CAD build for the part. Positions are in the model's coordinates, mm. A direction names the side the tool comes from. Coordinates: 2 decimals unless noted, no trailing zeros. Loops run counter-clockwise (first coordinate to the right, second up) from the corner with the lowest first, then second, coordinate; pieces in that order, holes last.
1) Which spindle directions (+Z, -Z, +X, -X, +Y, -Y) get a long thin tool onto all of the face, cutting with end or side? Do faces 1 (the flat face through (-1, -4, 1)), 2 (the cylindrical face through (-50.56, -3.26, 22.64)), 3 (the cylindrical face through (23.4, 1, -77.3)). Say none if no direction does.
2) Wall check: line 1 along X through (y, z) = (61.9, 87.42); line 2 along Z through (x, y) = (-12.5, 18.5); line 3 along Z through (x, y) = (-86.5, 63.55). Give the ranges that are in metal, low to high.
3) Pin check, flat tips, straight feed: pin 1 Ø0.8 at (x, z) = (-57, -70) entering from +Y; pin 2 Ø0.8 at (x, z) = (-25, -25.5) entering from -Y; pin 3 Ø0.6 at (y, z) = (28.5, -92) entering from -X. Stop position of each tip, or through.
4) Saw through at A-A, the plane y = 51. Write the cut outline in (x, z).
5) Saw through at B-B, the plane x = -4.5. Write the cut outline in (y, z).
6) Saw through at D-D, the plane x = 38.5. Write the cut outline in (y, z).
7) Two-plate mould, pull along Z, no slides. Class faces 4 (the flat face through (-1, 39, -92.92)), 5 (the cylindrical face through (-89.15, 30.98, 89.91)), 6 (the flat face through (86, 33, 83.92)): +Z half, -Z half, draft (parallel to the pull), parting line (faces both ways), or undercut.
8) Saw through at C-C, the plane z = 45. Write the cut outline in (x, y), and give its area (3 significant figures).
```python
from build123d import *

# Parameters (mm, degrees)
SKETCH1_W           = 184
SKETCH1_H           = 185.84
SKETCH1_W_2         = 180
SKETCH1_H_2         = 181.84
SKETCH1_W_3         = 7
SKETCH1_H_3         = 7
BOSS_EXTRUDE1_DEPTH = 65
SKETCH2_W           = 184
SKETCH2_H           = 185.84
BOSS_EXTRUDE2_DEPTH = 4
CUT_EXTRUDE1_REACH  = 187.84
SKETCH3_W           = 21.03
SKETCH3_H           = 16.02
CUT_EXTRUDE4_REACH  = 186
SKETCH4_R           = 1.75
SKETCH4_R_2         = 8.065
SKETCH4_W           = 4.5
SKETCH4_H           = 8.3
CUT_EXTRUDE3_REACH  = 187.84
SKETCH6_W           = 8.3
SKETCH6_H           = 4.5
SKETCH6_W_2         = 21.85
SKETCH6_H_2         = 30.2
SKETCH8_R           = 3.4
SKETCH8_R_2         = 1.4
SKETCH8_R_3         = 2.9
SKETCH8_R_4         = 0.9
BOSS_EXTRUDE3_DEPTH = 2
SKETCH8_3_R         = 2.14
BOSS_EXTRUDE4_DEPTH = 4
CUT_EXTRUDE5_REACH  = 6
SKETCH8_4_R         = 1.25
SKETCH9_R           = 2.25
CUT_EXTRUDE6_DEPTH  = 1.5
SKETCH10_R          = 1.4
CUT_EXTRUDE7_DEPTH  = 4
FILLET1_R           = 10
FILLET2_R           = 2
SKETCH11_R          = 1.4
CUT_EXTRUDE8_DEPTH  = 2.5


with BuildPart() as part:
    # Sketch1 → Boss-Extrude1 (new body)
    with BuildSketch(Plane(origin=(0, 0, 0), x_dir=(1, 0, 0), z_dir=(0, 1, 0))):
        Rectangle(SKETCH1_W, SKETCH1_H)
        Rectangle(SKETCH1_W_2, SKETCH1_H_2, mode=Mode.SUBTRACT)
        with Locations((-86.5, 87.42)):
            Rectangle(SKETCH1_W_3, SKETCH1_H_3)
        with Locations((86.5, 87.42)):
            Rectangle(SKETCH1_W_3, SKETCH1_H_3)
        with Locations((-86.5, -87.42)):
            Rectangle(SKETCH1_W_3, SKETCH1_H_3)
        with Locations((86.5, -87.42)):
            Rectangle(SKETCH1_W_3, SKETCH1_H_3)
    extrude(amount=BOSS_EXTRUDE1_DEPTH)

    # Sketch2 → Boss-Extrude2 (add)
    with BuildSketch(Plane.XZ):
        Rectangle(SKETCH2_W, SKETCH2_H)
    extrude(amount=BOSS_EXTRUDE2_DEPTH)

    # Sketch3 → Cut-Extrude1 (cut, up to next)
    with BuildSketch(Plane(origin=(0, 0, -92.92), x_dir=(-1, 0, 0), z_dir=(0, 0, -1)), mode=Mode.PRIVATE) as cut_extrude1_sk1:
        with Locations((0, 30.5)):
            Rectangle(SKETCH3_W, SKETCH3_H)
    cut_extrude1_tool1 = extrude(cut_extrude1_sk1.sketch, amount=-CUT_EXTRUDE1_REACH, mode=Mode.PRIVATE) & part.part
    add(cut_extrude1_tool1.solids().sort_by_distance((0, 30.5, -92.92))[0], mode=Mode.SUBTRACT)

    # Sketch4 → Cut-Extrude4 (cut, up to next)
    with BuildSketch(Plane(origin=(92, 0, 0), x_dir=(0, 0, -1), z_dir=(1, 0, 0)), mode=Mode.PRIVATE) as cut_extrude4_sk1:
        with Locations((-54.360232663, 46.940232663)):
            Circle(SKETCH4_R)
    cut_extrude4_tool1 = extrude(cut_extrude4_sk1.sketch, amount=-CUT_EXTRUDE4_REACH, mode=Mode.PRIVATE) & part.part
    add(cut_extrude4_tool1.solids().sort_by_distance((92, 46.940233, 54.360233))[0], mode=Mode.SUBTRACT)
    # Sketch4 → Cut-Extrude4 (cut, up to next)
    with BuildSketch(Plane(origin=(92, 0, 0), x_dir=(0, 0, -1), z_dir=(1, 0, 0)), mode=Mode.PRIVATE) as cut_extrude4_sk2:
        with Locations((-21.479767337, 14.059767337)):
            Circle(SKETCH4_R)
    cut_extrude4_tool2 = extrude(cut_extrude4_sk2.sketch, amount=-CUT_EXTRUDE4_REACH, mode=Mode.PRIVATE) & part.part
    add(cut_extrude4_tool2.solids().sort_by_distance((92, 14.059767, 21.479767))[0], mode=Mode.SUBTRACT)
    # Sketch4 → Cut-Extrude4 (cut, up to next)
    with BuildSketch(Plane(origin=(92, 0, 0), x_dir=(0, 0, -1), z_dir=(1, 0, 0)), mode=Mode.PRIVATE) as cut_extrude4_sk3:
        with Locations((52.92, 30.5)):
            Circle(SKETCH4_R_2)
    cut_extrude4_tool3 = extrude(cut_extrude4_sk3.sketch, amount=-CUT_EXTRUDE4_REACH, mode=Mode.PRIVATE) & part.part
    add(cut_extrude4_tool3.solids().sort_by_distance((92, 30.5, -52.92))[0], mode=Mode.SUBTRACT)
    # Sketch4 → Cut-Extrude4 (cut, up to next)
    with BuildSketch(Plane(origin=(92, 0, 0), x_dir=(0, 0, -1), z_dir=(1, 0, 0)), mode=Mode.PRIVATE) as cut_extrude4_sk4:
        with Locations((-71.17, 30.5)):
            Rectangle(SKETCH4_W, SKETCH4_H)
    cut_extrude4_tool4 = extrude(cut_extrude4_sk4.sketch, amount=-CUT_EXTRUDE4_REACH, mode=Mode.PRIVATE) & part.part
    add(cut_extrude4_tool4.solids().sort_by_distance((92, 30.5, 71.17))[0], mode=Mode.SUBTRACT)

    # Sketch6 → Cut-Extrude3 (cut, up to next)
    with BuildSketch(Plane.XY.offset(92.92), mode=Mode.PRIVATE) as cut_extrude3_sk1:
        with Locations((-41, 30.5)):
            Rectangle(SKETCH6_W, SKETCH6_H)
    cut_extrude3_tool1 = extrude(cut_extrude3_sk1.sketch, amount=-CUT_EXTRUDE3_REACH, mode=Mode.PRIVATE) & part.part
    add(cut_extrude3_tool1.solids().sort_by_distance((-41, 30.5, 92.92))[0], mode=Mode.SUBTRACT)
    # Sketch6 → Cut-Extrude3 (cut, up to next)
    with BuildSketch(Plane.XY.offset(92.92), mode=Mode.PRIVATE) as cut_extrude3_sk2:
        with Locations((-66.075, 30.5)):
            Rectangle(SKETCH6_W_2, SKETCH6_H_2)
    cut_extrude3_tool2 = extrude(cut_extrude3_sk2.sketch, amount=-CUT_EXTRUDE3_REACH, mode=Mode.PRIVATE) & part.part
    add(cut_extrude3_tool2.solids().sort_by_distance((-66.075, 30.5, 92.92))[0], mode=Mode.SUBTRACT)

    # Sketch8 → Boss-Extrude3 (add)
    with BuildSketch(Plane(origin=(0, 0, 0), x_dir=(1, 0, 0), z_dir=(0, 1, 0))):
        Polygon((-73.69124321, 46.82), (-80.626004845, 46.82), (-80.626004845, 39.885238365), (-82.626004845, 39.885238365), (-82.626004845, 48.82), (-73.69124321, 48.82), align=None)
        with Locations((-56.451004845, 69.7)):
            Circle(SKETCH8_R)
        with Locations((-56.451004845, 69.7)):
            Circle(SKETCH8_R_2, mode=Mode.SUBTRACT)
        with Locations((-25.911004845, 54.52)):
            Circle(SKETCH8_R)
        with Locations((-25.911004845, 54.52)):
            Circle(SKETCH8_R_2, mode=Mode.SUBTRACT)
        with Locations((23.733995155, 74.42)):
            Circle(SKETCH8_R_3)
        with Locations((23.733995155, 74.42)):
            Circle(SKETCH8_R_4, mode=Mode.SUBTRACT)
        with Locations((72.236687484, 26.922654466)):
            Circle(SKETCH8_R_3)
        with Locations((72.236687484, 26.922654466)):
            Circle(SKETCH8_R_4, mode=Mode.SUBTRACT)
        Polygon((0.273995155, 6.62), (-8.660766481, 6.62), (-8.660766481, 8.62), (-1.726004845, 8.62), (-1.726004845, 15.554761635), (0.273995155, 15.554761635), align=None)
    extrude(amount=BOSS_EXTRUDE3_DEPTH)

    # Sketch8_3 → Boss-Extrude4 (add)
    with BuildSketch(Plane(origin=(0, 0, 0), x_dir=(1, 0, 0), z_dir=(0, 1, 0))):
        with Locations((57.383995155, -6.52)):
            Circle(SKETCH8_3_R)
        with BuildLine():
            Line((59.523995155, -54.01), (59.523995155, -56.01))
            ThreePointArc((59.523995155, -56.01), (57.383995155, -58.15), (55.243995155, -56.01))
            Line((55.243995155, -56.01), (55.243995155, -54.01))
            ThreePointArc((55.243995155, -54.01), (57.383995155, -51.87), (59.523995155, -54.01))
        make_face()
    extrude(amount=BOSS_EXTRUDE4_DEPTH)

    # Sketch8_4 → Cut-Extrude5 (cut, up to next)
    with BuildSketch(Plane(origin=(0, 0, 0), x_dir=(1, 0, 0), z_dir=(0, 1, 0)), mode=Mode.PRIVATE) as cut_extrude5_sk1:
        with Locations((-48.776004845, -24.01)):
            Circle(SKETCH8_4_R)
    cut_extrude5_tool1 = extrude(cut_extrude5_sk1.sketch, amount=-CUT_EXTRUDE5_REACH, mode=Mode.PRIVATE) & part.part
    add(cut_extrude5_tool1.solids().sort_by_distance((-48.776005, 0, 24.01))[0], mode=Mode.SUBTRACT)
    # Sketch8_4 → Cut-Extrude5 (cut, up to next)
    with BuildSketch(Plane(origin=(0, 0, 0), x_dir=(1, 0, 0), z_dir=(0, 1, 0)), mode=Mode.PRIVATE) as cut_extrude5_sk2:
        with Locations((-12.616004845, -51.23)):
            Circle(SKETCH8_4_R)
    cut_extrude5_tool2 = extrude(cut_extrude5_sk2.sketch, amount=-CUT_EXTRUDE5_REACH, mode=Mode.PRIVATE) & part.part
    add(cut_extrude5_tool2.solids().sort_by_distance((-12.616005, 0, 51.23))[0], mode=Mode.SUBTRACT)

    # Sketch9 → Cut-Extrude6 (cut)
    with BuildSketch(Plane.XZ.offset(4)):
        with Locations((-12.616004845, 51.23)):
            Circle(SKETCH9_R)
        with Locations((-48.776004845, 24.01)):
            Circle(SKETCH9_R)
    extrude(amount=-CUT_EXTRUDE6_DEPTH, mode=Mode.SUBTRACT)

    # Sketch10 → Cut-Extrude7 (cut)
    with BuildSketch(Plane(origin=(0, 65, 0), x_dir=(1, 0, 0), z_dir=(0, 1, 0))):
        with Locations((-86.5, 87.42)):
            Circle(SKETCH10_R)
        with Locations((86.5, 87.42)):
            Circle(SKETCH10_R)
        with Locations((86.5, -87.42)):
            Circle(SKETCH10_R)
        with Locations((-86.5, -87.42)):
            Circle(SKETCH10_R)
    extrude(amount=-CUT_EXTRUDE7_DEPTH, mode=Mode.SUBTRACT)

    # Fillet1
    fillet1_edges = [part.edges().sort_by_distance(p)[0] for p in [
        (92, 30.5, -92.92),
        (92, 30.5, 92.92),
        (-92, 30.5, 92.92),
        (-92, 30.5, -92.92),
    ]]
    fillet(fillet1_edges, radius=FILLET1_R)

    # Fillet2
    fillet2_edges = [part.edges().sort_by_distance(p)[0] for p in [
        (0, 0, -90.92),
        (-90, 0, 0),
        (0, 0, 90.92),
        (90, 0, 0),
        (-83, 0, -87.42),
        (-86.5, 0, -83.92),
        (83, 0, -87.42),
        (86.5, 0, -83.92),
        (-83, 0, 87.42),
        (-86.5, 0, 83.92),
        (83, 0, 87.42),
        (86.5, 0, 83.92),
    ]]
    fillet(fillet2_edges, radius=FILLET2_R)

    # Sketch11 → Cut-Extrude8 (cut)
    with BuildSketch(Plane.XZ.offset(4)):
        with Locations((25, -25)):
            Circle(SKETCH11_R)
        with Locations((-25, -25)):
            Circle(SKETCH11_R)
        with Locations((25, 25)):
            Circle(SKETCH11_R)
        with Locations((-25, 25)):
            Circle(SKETCH11_R)
    extrude(amount=-CUT_EXTRUDE8_DEPTH, mode=Mode.SUBTRACT)


solid = part.part
```
Data:
1. face 1: +Z, -Z, +X, -X, -Y
1. face 2: -Y
1. face 3: +Y
2. line 1: x = -90.93 to -87.9, -85.1 to -83, 83 to 85.1, 87.9 to 90.93
2. line 2: z = -92.92 to -90.92, 90.92 to 92.92
2. line 3: z = -91.85 to -88.82, -86.02 to -83.92, 83.92 to 86.02, 88.82 to 91.85
3. pin 1: stops at y = 0
3. pin 2: stops at y = -1.5
3. pin 3: stops at x = -86.79
4. outline: (-92, -82.92) arc R10 ccw to (-82, -92.92) - (82, -92.92) arc R10 ccw to (92, -82.92) - (92, 82.92) arc R10 ccw to (82, 92.92) - (-82, 92.92) arc R10 ccw to (-92, 82.92) - close; hole (-90, -83.92) - (-83, -83.92) - (-83, -90.92) - (83, -90.92) - (83, -83.92) - (90, -83.92) - (90, 83.92) - (83, 83.92) - (83, 90.92) - (-83, 90.92) - (-83, 83.92) - (-90, 83.92) - close
5. outline: (-4, -92.92) - (22.49, -92.92) - (22.49, -90.92) - (2, -90.92) arc R2 cw to (0, -88.92) - (0, -8.62) - (2, -8.62) - (2, -6.62) - (0, -6.62) - (0, 88.92) arc R2 cw to (2, 90.92) - (65, 90.92) - (65, 92.92) - (-4, 92.92) - close; (38.51, -92.92) - (65, -92.92) - (65, -90.92) - (38.51, -90.92) - close
6. outline: (-4, -92.92) - (65, -92.92) - (65, -90.92) - (2, -90.92) arc R2 cw to (0, -88.92) - (0, 88.92) arc R2 cw to (2, 90.92) - (65, 90.92) - (65, 92.92) - (-4, 92.92) - close
7. face 4: -Z half
7. face 5: +Z half
7. face 6: undercut
8. outline: (-92, -4) - (92, -4) - (92, 65) - (90, 65) - (90, 2) arc R2 cw to (88, 0) - (-88, 0) arc R2 cw to (-90, 2) - (-90, 65) - (-92, 65) - close
8. area: 998 mm2
